Check sheet for the modelled part. Datum: model origin and axes. Units: mm. Give positions to 0.01 mm unless a question says otherwise; leave off trailing zeros. Write each loop counter-clockwise with the first axis right and the second up, starting at its lowest first coordinate (ties: lowest second). Pieces come first, ordered by that corner, then holes. Notation, with made-up numbers: M 69.25,39 L 90.25,39 A4 cw 90.25,44 Z; hole C 69.25,4 d1. An arc over 180 degrees is marked long. One line per item, written item: value. Start each with the question number.
from build123d import *

# Parameters (mm, degrees)
SKETCH1_R           = 15
BOSS_EXTRUDE1_DEPTH = 138.051909
SKETCH2_R           = 10.65749531
CUT_EXTRUDE1_DEPTH  = 140.672221929
CHAMFER1_SIZE       = 2.91936


with BuildPart() as part:
    # Sketch1 → Boss-Extrude1 (new body)
    with BuildSketch(Plane(origin=(0, 0, 0), x_dir=(1, 0, 0), z_dir=(0, 1, 0))):
        with Locations(Location((0, 0, 0), (0, 0, 90))):
            Circle(SKETCH1_R)
    extrude(amount=BOSS_EXTRUDE1_DEPTH)

    # Sketch2 → Cut-Extrude1 (cut, through all)
    with BuildSketch(Plane(origin=(0, 0, 0), x_dir=(1, 0, 0), z_dir=(0, 1, 0))):
        with Locations(Location((0, 0, 0), (0, 0, 90))):
            Circle(SKETCH2_R)
    extrude(amount=CUT_EXTRUDE1_DEPTH, mode=Mode.SUBTRACT)

    # Chamfer1
    chamfer1_edges = [part.edges().sort_by_distance(p)[0] for p in [
        (0, 0, 15),
        (0, 138.051909, 15),
    ]]
    chamfer(chamfer1_edges, length=CHAMFER1_SIZE)


solid = part.part
1) Cross-section at B-B (z = 0). Record the boundary of the cut face in (x, y).
2) Gauge pin test, flat ends, axial feed: pin 1 (8 mm diameter, centred on y = 110.5, z = -2.5, fed in from -X); pin 2 (1 mm diameter, centred on x = 3.5, y = 77, fed in from +Z); pin 3 (12 mm diameter, centred on x = 3.5, z = 0.5, fed in from +Y); pin 4 (1 mm diameter, centred on y = 29.5, z = -6, fed in from +X). Record the tip position at first contact, or that the pin passes through.
3) Cross-section at C-C (y = 18). Record the boundary of the cut face in (x, z) (1 decimal), plus the area to 3 significant figures.
4) Material ranges on L1, parallel to X at y = 33.5, z = 0; L2, parallel to X at y = 44, z = 1.5; L3, parallel to Z at x = 1.75, y = 8, recorded low to high. Write a range as from..to.
5) Draft check along X on faces 1 (the flat face through (11, 0, 0)), 2 (the cylindrical face through (-8.986, 68.06, -5.729)), 3 (the conical face through (-3.671, 0.142, -11.658)). Enter one of: released by +X, released by -X, zero draft, split by the parting line, or undercut.
6) Cross-section at A-A (x = 0). Record the boundary of the cut face in (y, z).
Data:
1. outline: M -15,2.92 L -12.08,0 L -10.66,0 L -10.66,138.05 L -12.08,138.05 L -15,135.13 Z; M 10.66,0 L 12.08,0 L 15,2.92 L 15,135.13 L 12.08,138.05 L 10.66,138.05 Z
2. pin 1: stops at x = -15
2. pin 2: stops at z = 14.7
2. pin 3: passes through
2. pin 4: stops at x = 13.96
3. outline: C 0,0 d30; hole C 0,0 d21.3
3. area: 350 mm2
4. L1: x = -15..-10.66, 10.66..15
4. L2: x = -14.92..-10.55, 10.55..14.92
4. L3: z = -14.9..-10.51, 10.51..14.9
5. face 1: zero draft
5. face 2: undercut
5. face 3: split by the parting line
6. outline: M 0,-12.08 L 2.92,-15 L 135.13,-15 L 138.05,-12.08 L 138.05,-10.66 L 0,-10.66 Z; M 0,10.66 L 138.05,10.66 L 138.05,12.08 L 135.13,15 L 2.92,15 L 0,12.08 Z
